from build123d import *

# Parameters (mm, degrees)
SKETCH_1_R          = 1.4
EXTRUDE_1_DEPTH     = 2
CUT_EXTRUDE_1_DEPTH = 1


with BuildPart() as part:
    # Эскиз1 → Бобышка-Вытянуть1 (new body)
    with BuildSketch(Plane.XY):
        with BuildLine():
            Line((78, 0), (89, 0))
            ThreePointArc((89, 0), (89.707106781, 0.292893219), (90, 1))
            Line((90, 1), (90, 12))
            Line((90, 12), (90, 29))
            ThreePointArc((90, 29), (89.707106781, 29.707106781), (89, 30))
            Line((89, 30), (1, 30))
            ThreePointArc((1, 30), (0.292893219, 29.707106781), (0, 29))
            Line((0, 29), (0, 1))
            ThreePointArc((0, 1), (0.292893219, 0.292893219), (1, 0))
            Line((1, 0), (60.966683233, 0))
            Line((60.966683233, 0), (78, 0))
        make_face()
        with Locations((3, 3)):
            Circle(SKETCH_1_R, mode=Mode.SUBTRACT)
        with Locations((3, 25)):
            Circle(SKETCH_1_R, mode=Mode.SUBTRACT)
        with Locations((87, 25)):
            Circle(SKETCH_1_R, mode=Mode.SUBTRACT)
        with Locations((77, 3)):
            Circle(SKETCH_1_R, mode=Mode.SUBTRACT)
    extrude(amount=EXTRUDE_1_DEPTH)

    # Эскиз2 → Вырез-Вытянуть1 (cut)
    with BuildSketch(Plane(origin=(0, 0, 0), x_dir=(-1, 0, 0), z_dir=(0, 0, -1))):
        with BuildLine():
            Line((-82, 28), (-8, 28))
            ThreePointArc((-8, 28), (-7.292893219, 27.707106781), (-7, 27))
            Line((-7, 27), (-7, 23))
            ThreePointArc((-7, 23), (-6.707106781, 22.292893219), (-6, 22))
            Line((-6, 22), (-3, 22))
            ThreePointArc((-3, 22), (-2.292893219, 21.707106781), (-2, 21))
            Line((-2, 21), (-2, 8))
            ThreePointArc((-2, 8), (-2.292893219, 7.292893219), (-3, 7))
            Line((-3, 7), (-6, 7))
            ThreePointArc((-6, 7), (-6.707106781, 6.707106781), (-7, 6))
            Line((-7, 6), (-7, 3))
            ThreePointArc((-7, 3), (-7.292893219, 2.292893219), (-8, 2))
            Line((-8, 2), (-72, 2))
            ThreePointArc((-72, 2), (-72.707106781, 2.292893219), (-73, 3))
            Line((-73, 3), (-73, 6))
            ThreePointArc((-73, 6), (-73.292893219, 6.707106781), (-74, 7))
            Line((-74, 7), (-78.5, 7))
            ThreePointArc((-78.5, 7), (-79.207106781, 6.707106781), (-79.5, 6))
            Line((-79.5, 6), (-79.5, 2.5))
            ThreePointArc((-79.5, 2.5), (-79.792893219, 1.792893219), (-80.5, 1.5))
            Line((-80.5, 1.5), (-87.5, 1.5))
            ThreePointArc((-87.5, 1.5), (-88.207106781, 1.792893219), (-88.5, 2.5))
            Line((-88.5, 2.5), (-88.5, 21))
            ThreePointArc((-88.5, 21), (-88.207106781, 21.707106781), (-87.5, 22))
            Line((-87.5, 22), (-84, 22))
            ThreePointArc((-84, 22), (-83.292893219, 22.292893219), (-83, 23))
            Line((-83, 23), (-83, 27))
            ThreePointArc((-83, 27), (-82.707106781, 27.707106781), (-82, 28))
        make_face()
    extrude(amount=-CUT_EXTRUDE_1_DEPTH, mode=Mode.SUBTRACT)


solid = part.part
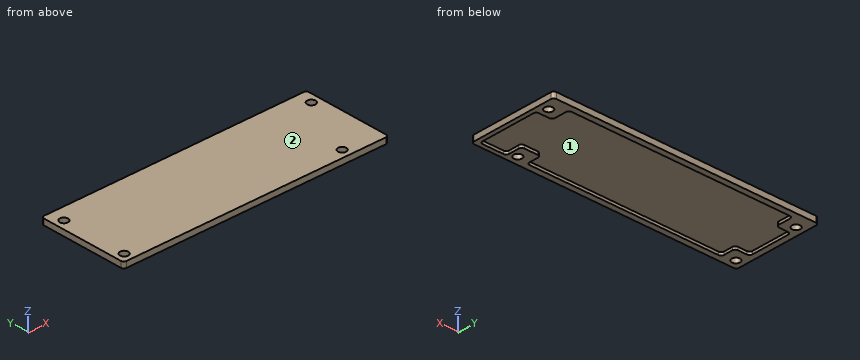
Input: part model. Units: mm. Frame: model coordinates. Face numbers are marked on the shaded views. Coordinates: 2 decimals unless noted, no trailing zeros. Loops run counter-clockwise (first coordinate to the right, second up) from the corner with the lowest first, then second, coordinate; pieces in that order, holes last. Notation, with made-up numbers: (-3.5, -35.5) - (27.5, -35.5) arc R30 cw to (27.5, -12.5) - close; hole circle Ø7 at (0, 6). An arc over 180 degrees is marked (long way). Answer in a Markdown table with one row per item. Add a question column.
Item 1: Contact query for flat-ended pins moving along their axis: P1, Ø2, axis at x = 3, y = 3, coming from the -Z side; P2, Ø3.5, axis at x = 77, y = 3, coming from the -Z side. Output: stop coordinate, or through.
Item 2: Section query B-B on x = 77. Return the cut outline in (y, z).
Item 3: Section query C-C on x = 36.5. Return the cut outline in (y, z).
Item 4: Section query D-D on z = 0.3. State how many separate pieces and enclosed holes the cut face has, then the cut area to 3 significant figures.
Item 5: Section query A-A on y = 25. Return the cut outline in (x, z).
Item 6: Mould query, pull axis Y, two halves, no side actions, for the marked faces 1 and 2. Classes: released by +Y, released by -Y, zero draft, split by the parting line, or undercut.
Item 7: Line query: line 1 along Y through (x, z) = (3, 0.65); line 2 along X through (y, z) = (6, 0.5); line 3 along Y through (x, z) = (3, 1.1). Output: solid intervals per line, ascending. Write a range as [from, to].
Recorded:
| question | item | result |
|---|---|---|
| 1 | P1 | through |
| 1 | P2 | z = 0 |
| 2 | outline | (0, 0) - (1.6, 0) - (1.6, 2) - (0, 2) - close; (4.4, 0) - (7, 0) - (7, 1) - (28, 1) - (28, 0) - (30, 0) - (30, 2) - (4.4, 2) - close |
| 3 | outline | (0, 0) - (2, 0) - (2, 1) - (28, 1) - (28, 0) - (30, 0) - (30, 2) - (0, 2) - close |
| 4 | separate pieces | 1 |
| 4 | enclosed holes | 5 |
| 4 | area | 542 mm^2 |
| 5 | outline | (0, 0) - (1.6, 0) - (1.6, 2) - (0, 2) - close; (4.4, 0) - (7, 0) - (7, 1) - (83, 1) - (83, 0) - (85.6, 0) - (85.6, 2) - (4.4, 2) - close; (88.4, 0) - (90, 0) - (90, 2) - (88.4, 2) - close |
| 6 | face 1 | undercut |
| 6 | face 2 | zero draft |
| 7 | line 1 | [0, 1.6], [4.4, 7], [22, 23.6], [26.4, 30] |
| 7 | line 2 | [0, 7], [73, 79.5], [88.5, 90] |
| 7 | line 3 | [0, 1.6], [4.4, 23.6], [26.4, 30] |
